For this review, take the finished solid that the model builds, in its own axes (mm). Face numbers are marked on the shaded views. A direction names the side the tool comes from. Coordinates: 2 decimals unless noted, no trailing zeros. Loops run counter-clockwise (first coordinate to the right, second up) from the corner with the lowest first, then second, coordinate; pieces in that order, holes last. Notation, with made-up numbers: (54, 4.25) - (66, 4.25) arc R24 ccw to (66, 41.25) - close; hole circle Ø6 at (2, 65.25). An arc over 180 degrees is marked (long way). Answer as a JSON object with one key per item and string values. Group by question number.
Item 1: We need section D-D (z = 15.5). Give the boundary of the cut face in (x, y), then the cut area to 3 significant figures.
Item 2: We need section A-A (z = 2.5). Give the boundary of the cut face in (x, y), then the cut area to 3 significant figures.
Item 3: To check wall thickness, follow line 1 (X direction, y = 0.4, z = 0); line 2 (X direction, y = 5.3, z = -1). State the ranges of each line that lie inside material, in increasing order.
Item 4: Tool access review of the marked faces 1 and 2: name each direction out of +Z, -Z, +X, -X, +Y, -Y from which nothing blocks a thin tool from reaching the whole face with its end or side.
Item 5: We need section C-C (y = 3.65). State how many separate pieces and enclosed holes the cut face has, then the cut area to 3 significant figures.
Item 6: Clearance check with flat-ended pins moving along their axes: pin 1 (5.5 mm diameter, centred on x = 25, z = 15.5, fed in from +Y); pin 2 (3 mm diameter, centred on x = -24, z = 15, fed in from -Y); pin 3 (2 mm diameter, centred on x = 25, z = -15.5, fed in from +Y). State where each tip first meets the part, or that it passes through.
Item 7: We need section B-B (x = 15.5). Give the boundary of the cut face in (y, z), then the cut area to 3 significant figures.
from build123d import *

# Parameters (mm, degrees)
SKETCH_1_W                           = 57
SKETCH_1_H                           = 57
EXTRUDE_1_DEPTH                      = 5
SKETCH_2_R                           = 25.1
CUT_EXTRUDE_1_DEPTH                  = 3
CUT_EXTRUDE_5_DEPTH                  = 41.416580756
CUT_EXTRUDE_5_DEPTH_BACK             = 41.416580756
SKETCH_8_R                           = 23.5
SKETCH_3_R                           = 2.5
SKETCH_3_R_2                         = 1.7
CUT_EXTRUDE_2_DEPTH                  = 41.614036982
CUT_EXTRUDE_4_DEPTH                  = 2.5
EXTRUDE_2_DEPTH                      = 1
CHAMFER_1_SIZE                       = 0.2
CUT_EXTRUDE_3_DEPTH                  = 1.1
PATTERN_CIRCULAR_1_COUNT             = 4
CHAMFER_1_OF_PATTERN_CIRCULAR_1_SIZE = 0.2
FILLET_1_R                           = 5


with BuildPart() as part:
    # 草图1 → 凸台-拉伸1 (new body)
    with BuildSketch(Plane(origin=(0, 0, 0), x_dir=(1, 0, 0), z_dir=(0, 1, 0))):
        Rectangle(SKETCH_1_W, SKETCH_1_H)
    extrude(amount=EXTRUDE_1_DEPTH)

    # 草图2 → 切除-拉伸1 (cut)
    with BuildSketch(Plane(origin=(0, 5, 0), x_dir=(1, 0, 0), z_dir=(0, 1, 0))):
        with Locations(Location((0, 0, 0), (0, 0, 270))):
            Circle(SKETCH_2_R)
    extrude(amount=-CUT_EXTRUDE_1_DEPTH, mode=Mode.SUBTRACT)

    # 草图8 → 切除-拉伸5 (cut, two sides: drawn at the far end of the back side and taken through both)
    with BuildSketch(Plane(origin=(0, 2, 0), x_dir=(1, 0, 0), z_dir=(0, 1, 0)).offset(-CUT_EXTRUDE_5_DEPTH_BACK)):
        with Locations(Location((0, 0, 0), (0, 0, 270))):
            Circle(SKETCH_8_R)
    extrude(amount=CUT_EXTRUDE_5_DEPTH + CUT_EXTRUDE_5_DEPTH_BACK, mode=Mode.SUBTRACT)

    # 草图3 → 切除-拉伸2 (cut, through all)
    with BuildSketch(Plane(origin=(0, 5, 0), x_dir=(1, 0, 0), z_dir=(0, 1, 0))):
        with Locations(Location((23.5, 23.5, 0), (0, 0, 270))):
            Circle(SKETCH_3_R)
        with Locations(Location((25, 15.5, 0), (0, 0, 270))):
            Circle(SKETCH_3_R_2)
        with Locations(Location((15.5, 25, 0), (0, 0, 90))):
            Circle(SKETCH_3_R_2)
    cut_extrude_2 = extrude(amount=-CUT_EXTRUDE_2_DEPTH, mode=Mode.SUBTRACT)

    # 草图7 → 切除-拉伸4 (cut)
    with BuildSketch(Plane.XZ):
        Polygon((27.75, -13.91228676), (25, -12.324573519), (22.25, -13.91228676), (22.25, -17.08771324), (25, -18.675426481), (27.75, -17.08771324), align=None)
    cut_extrude_4 = extrude(amount=-CUT_EXTRUDE_4_DEPTH, mode=Mode.SUBTRACT)

    # 草图4 → 凸台-拉伸2 (add)
    with BuildSketch(Plane(origin=(0, 5, 0), x_dir=(1, 0, 0), z_dir=(0, 1, 0))):
        Polygon((28.5, 11), (27.5, 10), (27.5, -10), (28.5, -11), align=None)
    extrude_2 = extrude(amount=EXTRUDE_2_DEPTH)

    # 倒角1
    chamfer_1_edges = [part.edges().sort_by_distance(p)[0] for p in [
        (27.5, 6, 0),
    ]]
    chamfer(chamfer_1_edges, length=CHAMFER_1_SIZE)

    # 草图5 → 切除-拉伸3 (cut)
    with BuildSketch(Plane.XZ):
        Polygon((28.5, 11.1), (27.5, 10.1), (27.5, -10.1), (28.5, -11.1), align=None)
    cut_extrude_3 = extrude(amount=-CUT_EXTRUDE_3_DEPTH, mode=Mode.SUBTRACT)

    # 阵列(圆周)1: 切除-拉伸2, 切除-拉伸4, 凸台-拉伸2, 切除-拉伸3 ×4 about axis
    pattern_circular_1_axis = Axis((0, 0, 0), (0, 1, 0))
    add([cut_extrude_2.rotate(pattern_circular_1_axis, i * 360 / PATTERN_CIRCULAR_1_COUNT) for i in range(1, PATTERN_CIRCULAR_1_COUNT)], mode=Mode.SUBTRACT)
    add([cut_extrude_4.rotate(pattern_circular_1_axis, i * 360 / PATTERN_CIRCULAR_1_COUNT) for i in range(1, PATTERN_CIRCULAR_1_COUNT)], mode=Mode.SUBTRACT)
    add([extrude_2.rotate(pattern_circular_1_axis, i * 360 / PATTERN_CIRCULAR_1_COUNT) for i in range(1, PATTERN_CIRCULAR_1_COUNT)])
    add([cut_extrude_3.rotate(pattern_circular_1_axis, i * 360 / PATTERN_CIRCULAR_1_COUNT) for i in range(1, PATTERN_CIRCULAR_1_COUNT)], mode=Mode.SUBTRACT)

    # 倒角1 of 阵列(圆周)1
    chamfer_1_of_pattern_circular_1_edges = [part.edges().sort_by_distance(p)[0] for p in [
        (0, 6, -27.5),
        (-27.5, 6, 0),
        (0, 6, 27.5),
    ]]
    chamfer(chamfer_1_of_pattern_circular_1_edges, length=CHAMFER_1_OF_PATTERN_CIRCULAR_1_SIZE)

    # 圆角1
    fillet_1_edges = [part.edges().sort_by_distance(p)[0] for p in [
        (28.5, 2.5, 28.5),
        (-28.5, 2.5, 28.5),
        (-28.5, 2.5, -28.5),
        (28.5, 2.5, -28.5),
    ]]
    fillet(fillet_1_edges, radius=FILLET_1_R)


solid = part.part
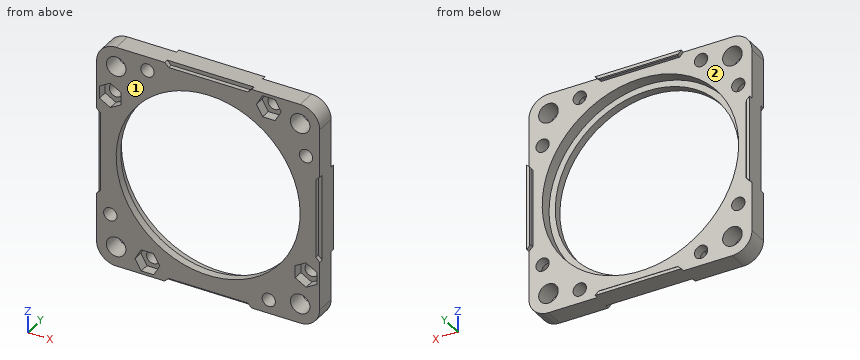
Check sheet entries:
{
 "1": {"outline": "(-28.5, 0) - (-27.75, 0) - (-27.75, 2.5) - (-26.7, 2.5) - (-26.7, 5) - (-28.5, 5) - close; (-23.3, 2.5) - (-22.25, 2.5) - (-22.25, 0) - (-17.66, 0) - (-17.66, 2) - (-19.74, 2) - (-19.74, 5) - (-23.3, 5) - close; (17.66, 0) - (23.3, 0) - (23.3, 5) - (19.74, 5) - (19.74, 2) - (17.66, 2) - close; (26.7, 0) - (28.5, 0) - (28.5, 5) - (26.7, 5) - close", "area": "56.6 mm2"},
 "2": {"outline": "(-28.5, 1.1) - (-27.5, 1.1) - (-27.5, 0) - (-23.37, 0) - (-23.37, 2) - (-24.98, 2) - (-24.98, 5) - (-27.5, 5) - (-27.5, 5.8) - (-27.7, 6) - (-28.5, 6) - close; (23.37, 0) - (27.5, 0) - (27.5, 1.1) - (28.5, 1.1) - (28.5, 6) - (27.7, 6) - (27.5, 5.8) - (27.5, 5) - (24.98, 5) - (24.98, 2) - (23.37, 2) - close", "area": "41.4 mm2"},
 "3": {"line 1": "x = -27.5 to -23.5, 23.5 to 27.5", "line 2": "x = -28.5 to -27.5, 27.5 to 28.5"},
 "4": {"face 1": "+Z, -Z, +X, -X, -Y", "face 2": "+Y"},
 "5": {"separate pieces": "1", "enclosed holes": "13", "area": "1,100 mm2"},
 "6": {"pin 1": "stops at y = 5", "pin 2": "stops at y = 2.5", "pin 3": "passes through"},
 "7": {"outline": "(0, -28.5) - (5, -28.5) - (5, -26.7) - (0, -26.7) - close; (0, -23.3) - (5, -23.3) - (5, -19.74) - (2, -19.74) - (2, -17.66) - (0, -17.66) - close; (0, 17.66) - (2, 17.66) - (2, 19.74) - (5, 19.74) - (5, 23.3) - (2.5, 23.3) - (2.5, 22.25) - (0, 22.25) - close; (0, 27.75) - (2.5, 27.75) - (2.5, 26.7) - (5, 26.7) - (5, 28.5) - (0, 28.5) - close", "area": "56.6 mm2"}
}
